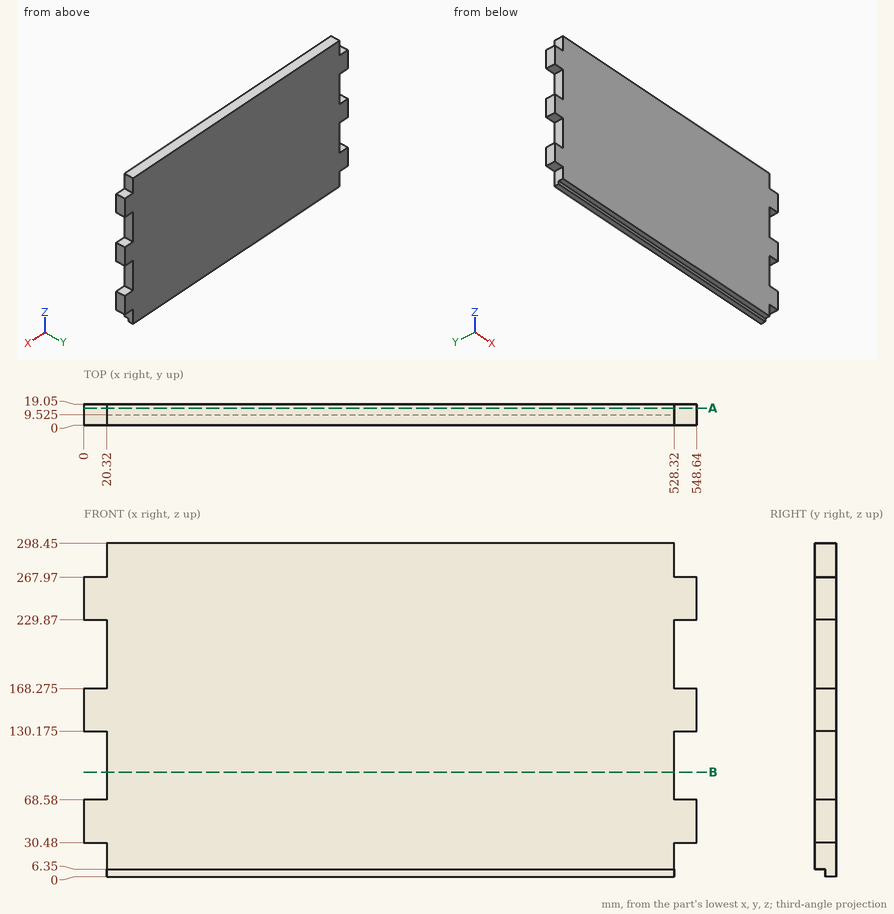
Input: dimensioned drawing with shaded views. Units: mm. Origin: part minimum x, y, z. Give positions to 0.01 mm unless a question says otherwise; leave off trailing zeros. Write each loop counter-clockwise with the first axis right and the second up, starting at its lowest first coordinate (ties: lowest second). Pieces come first, ordered by that corner, then holes.
1. Material intervals for line 1 along X through (y, z) = (8.5, 26); line 2 along Z through (x, y) = (80, 1.75), sorted ascending.
2. Section query B-B (z = 93.5). Return the cut outline in (x, y), then the cut area to 3 significant figures.
3. Section query A-A (y = 15.25). Return the cut outline in (x, z) (3 decimals).
4. First-contact query: pin 1 (9.5 mm diameter, centred on x = 541, y = 7, fed in from +Z); pin 2 (12 mm diameter, centred on x = 319, z = 197.5, fed in from -Y); pin 3 (9.5 mm diameter, centred on x = 13, y = 13.5, fed in from -Z); pin 4 (3 mm diameter, centred on x = 379, y = 6.5, fed in from -Z). Flat tips, straight axial feed; report the tip coordinate or a pass-through.
Output values:
1. line 1: x = 20.32 to 528.32
1. line 2: z = 6.35 to 298.45
2. outline: (20.32, 0) - (528.32, 0) - (528.32, 19.05) - (20.32, 19.05) - close
2. area: 9,680 mm2
3. outline: (0, 30.48) - (20.32, 30.48) - (20.32, 0) - (528.32, 0) - (528.32, 30.48) - (548.64, 30.48) - (548.64, 68.58) - (528.32, 68.58) - (528.32, 130.175) - (548.64, 130.175) - (548.64, 168.275) - (528.32, 168.275) - (528.32, 229.87) - (548.64, 229.87) - (548.64, 267.97) - (528.32, 267.97) - (528.32, 298.45) - (20.32, 298.45) - (20.32, 267.97) - (0, 267.97) - (0, 229.87) - (20.32, 229.87) - (20.32, 168.275) - (0, 168.275) - (0, 130.175) - (20.32, 130.175) - (20.32, 68.58) - (0, 68.58) - close
4. pin 1: stops at z = 267.97
4. pin 2: stops at y = 0
4. pin 3: stops at z = 30.48
4. pin 4: stops at z = 6.35
